Here's how the part is built. I have some questions about the finished solid (model axes, mm). A direction names the side the tool comes from. Coordinates: 2 decimals unless noted, no trailing zeros. Write each loop counter-clockwise with the first axis right and the second up, starting at its lowest first coordinate (ties: lowest second). Pieces come first, ordered by that corner, then holes.
```python
from build123d import *

# Parameters (mm, degrees)
F1_DEPTH = 6
F4_D     = 2.6
F5_D     = 2.6
F5_DEPTH = 9
F5_TIP   = 0.7811188047


with BuildPart() as f1:
    # F0 (on Right) → F1 (new body)
    with BuildSketch(Plane.YZ):
        Polygon((0, 8), (0, 0), (7, 0), (7, 1.6), (16, 1.6), (16, 13), (5, 13), align=None)
    extrude(amount=F1_DEPTH)

    # F4 (through all)
    with Locations(Plane.XY.offset(13)):
        with Locations((3, 11.5)):
            Hole(F4_D / 2)

    # F5
    with Locations(Plane.XZ):
        with Locations((3, 4)):
            Hole(F5_D / 2, depth=F5_DEPTH)
            with Locations((0, 0, -(F5_DEPTH + F5_TIP / 2))):  # 118° drill point
                Cone(0, F5_D / 2, F5_TIP, mode=Mode.SUBTRACT)


solid = f1.part
```
1) Imagine slicing it at A-A on y = 11.5. Please give me the cut outline in (x, z).
Values follow:
outline: (0, 1.6) - (1.7, 1.6) - (1.7, 13) - (0, 13) - close; (4.3, 1.6) - (6, 1.6) - (6, 13) - (4.3, 13) - close
2) I need wall thicknesses on probe 1 along Z at (x, y) = (3.1, 7.5); probe 2 along Y at (x, z) = (3, 6.75); probe 3 along X at (y, z) = (6.5, 4). Which ranges of each line are inside material? Lowest first, please.
Values follow:
probe 1: z = 1.6 to 2.7, 5.3 to 13
probe 2: y = 0 to 10.2, 12.8 to 16
probe 3: x = 0 to 1.7, 4.3 to 6
3) We'd pull the mould along Z, two halves only. Please class faces 1 (the face through (3.28, 4.56, 2.73)), 2 (the face through (3, 3, 0)), 3 (the face through (3.17, 12.79, 7.22)): pulls with the +Z half, pulls with the -Z half, needs draft (parallel to the pull), parting line crosses it, or undercut.
Values follow:
face 1: undercut
face 2: pulls with the -Z half
face 3: needs draft
4) Imagine slicing it at D-D on x = 5.45. Please give me the cut outline in (y, z).
Values follow:
outline: (0, 0) - (7, 0) - (7, 1.6) - (16, 1.6) - (16, 13) - (5, 13) - (0, 8) - close
5) Imagine slicing it at C-C on y = 3. Please give me the cut outline in (x, z), then the cut area to 3 significant figures.
Values follow:
outline: (0, 0) - (6, 0) - (6, 11) - (0, 11) - close; hole circle Ø2.6 at (3, 4)
area: 60.7 mm2
6) On a 3-axis mill with a long thin cutter (end or side, diameter ignored), from which of +Z, -Z, +X, -X, +Y, -Y can I reach the whole of each face in a straight line? I mean faces 4 (the face through (0, 8, 7)), 5 (the face through (3, 7, 1)). Say none if no direction works.
Values follow:
face 4: +Z, -Z, -X, +Y, -Y
face 5: -Z, +X, -X, +Y
7) Will this pin go through, and if not, where does the flat tip stop? pin 1 (1.6 mm diameter, centred on x = 3, z = 4, fed in from -Y).
Values follow:
pin 1: stops at y = 9.3
8) Imagine slicing it at B-B on z = 2.25. Please give me the cut outline in (x, y).
Values follow:
outline: (0, 0) - (6, 0) - (6, 16) - (0, 16) - close; hole circle Ø2.6 at (3, 11.5)
